```python
from build123d import *

# Parameters (mm, degrees)
SKETCH1_W           = 13
SKETCH1_H           = 10
BOSS_EXTRUDE1_DEPTH = 7.5
SKETCH2_R           = 2.5
CUT_EXTRUDE1_DEPTH  = 15
FILLET1_R           = 5
SKETCH3_W           = 46
SKETCH3_H           = 7
BOSS_EXTRUDE2_DEPTH = 5
SKETCH4_W           = 4
SKETCH4_H           = 7
BOSS_EXTRUDE3_DEPTH = 45
SKETCH5_W           = 5
SKETCH5_H           = 13
BOSS_EXTRUDE4_DEPTH = 30


with BuildPart() as part:
    # Sketch1 → Boss-Extrude1 (new, symmetric)
    with BuildSketch(Plane(origin=(0, 0, 0), x_dir=(0, 0, -1), z_dir=(1, 0, 0))):
        Rectangle(SKETCH1_W, SKETCH1_H)
    extrude(amount=BOSS_EXTRUDE1_DEPTH, both=True)

    # Sketch2 → Cut-Extrude1 (cut)
    with BuildSketch(Plane.XY.offset(6.5)):
        with Locations((-1.5, 0)):
            Circle(SKETCH2_R)
    extrude(amount=-CUT_EXTRUDE1_DEPTH, mode=Mode.SUBTRACT)

    # Fillet1
    fillet1_edges = [part.edges().sort_by_distance(p)[0] for p in [
        (-7.5, -5, 0),
        (-7.5, 5, 0),
    ]]
    fillet(fillet1_edges, radius=FILLET1_R - 0.0001)  # a hair under: the kernel refuses the full size

    # Sketch3 → Boss-Extrude2 (add)
    with BuildSketch(Plane(origin=(7.5, 0, 0), x_dir=(0, 0, -1), z_dir=(1, 0, 0))):
        Rectangle(SKETCH3_W, SKETCH3_H)
    extrude(amount=BOSS_EXTRUDE2_DEPTH)

    # Sketch4 → Boss-Extrude3 (add)
    with BuildSketch(Plane(origin=(12.5, 0, 0), x_dir=(0, 0, -1), z_dir=(1, 0, 0))):
        with Locations((-21, 0)):
            Rectangle(SKETCH4_W, SKETCH4_H)
        with Locations((21, 0)):
            Rectangle(SKETCH4_W, SKETCH4_H)
    extrude(amount=BOSS_EXTRUDE3_DEPTH)

    # Sketch5 → Boss-Extrude4 (add)
    with BuildSketch(Plane(origin=(0, 3.5, 0), x_dir=(1, 0, 0), z_dir=(0, 1, 0))):
        with Locations((10, 0)):
            Rectangle(SKETCH5_W, SKETCH5_H)
    boss_extrude4 = extrude(amount=BOSS_EXTRUDE4_DEPTH)

    # Mirror1: Boss-Extrude4 across plane
    add(boss_extrude4.mirror(Plane.ZX))


solid = part.part
```
Part model, mm, in its own coordinate system. A direction names the side the tool comes from. Round coordinates to 2 decimals unless told otherwise and drop trailing zeros. Write each loop counter-clockwise with the first axis right and the second up, starting at its lowest first coordinate (ties: lowest second). Pieces come first, ordered by that corner, then holes. Notation, with made-up numbers: M 82,89.25 L 97,89.25 A10 ccw 97,102.25 Z; hole C -17,10 d4. An arc over 180 degrees is marked long. One line per question, with ' | ' between items.
(1) Probe line 1 along Y through (x, z) = (-1.5, -3.5); line 2 along Z through (x, y) = (55.5, -1); line 3 along X through (y, z) = (22.5, -3). List the from-to ranges inside material, lowest first.
Answer key:
line 1: y = -5 to -2.5, 2.5 to 5 | line 2: z = -23 to -19, 19 to 23 | line 3: x = 7.5 to 12.5
(2) 3-axis set-ups, long thin cutter, end or side, ignore diameter. For faces 1 (the face through (7.5, 0, -15)), 2 (the face through (3, -5, 0)), 3 (the face through (7.5, 19, 0)), 4 (the face through (35, 0, -19)), 5 (the face through (25, 3.5, -20)): which of +Z, -Z, +X, -X, +Y, -Y reach the whole face in a straight line?
Answer key:
face 1: -Z, -X, +Y, -Y | face 2: +Z, -Z, -X, -Y | face 3: +Z, -Z, -X, +Y | face 4: +X, +Y, -Y | face 5: -Z, +X, -X, +Y
(3) Two-plate mould, pull along X, no slides. Class faces 6 (the face through (-6.07, 3.5, -0.09)), 7 (the face through (35, 0, 19)), 8 (the face through (-4, 0, 0)): released by +X, released by -X, zero draft, split by the parting line, or undercut.
Answer key:
face 6: released by -X | face 7: zero draft | face 8: undercut
(4) Saw through at A-A on x = -1.5. Write the cut outline in (y, z).
Answer key:
outline: M -5,-6.5 L -2.5,-6.5 L -2.5,6.5 L -5,6.5 Z; M 2.5,-6.5 L 5,-6.5 L 5,6.5 L 2.5,6.5 Z
(5) Saw through at C-C on z = -13.5. Write the cut outline in (x, y), then the cut area to 3 significant figures.
Answer key:
outline: M 7.5,-3.5 L 12.5,-3.5 L 12.5,3.5 L 7.5,3.5 Z | area: 35.0 mm^2
(6) Pin check, flat tips, straight feed: pin 1 (2 mm diameter, centred on y = 1.5, z = -11.5, fed in from -X); pin 2 (10 mm diameter, centred on x = 29.5, z = -15.5, fed in from -Y); pin 3 (22 mm diameter, centred on x = -2.5, y = 13.5, fed in from +Z). Stop position of each tip, or through.
Answer key:
pin 1: stops at x = 7.5 | pin 2: stops at y = -3.5 | pin 3: stops at z = 6.5
(7) Saw through at D-D on x = 32.5. Write the cut outline in (y, z), then the cut area to 3 significant figures.
Answer key:
outline: M -3.5,-23 L 3.5,-23 L 3.5,-19 L -3.5,-19 Z; M -3.5,19 L 3.5,19 L 3.5,23 L -3.5,23 Z | area: 56.0 mm^2
(8) Saw through at B-B on x = 9.5. Write the cut outline in (y, z).
Answer key:
outline: M -33.5,-6.5 L -3.5,-6.5 L -3.5,-23 L 3.5,-23 L 3.5,-6.5 L 33.5,-6.5 L 33.5,6.5 L 3.5,6.5 L 3.5,23 L -3.5,23 L -3.5,6.5 L -33.5,6.5 Z
